For this review, take the finished solid that the model builds, in its own axes (mm). A direction names the side the tool comes from. Give positions to 0.01 mm unless a question says otherwise; leave off trailing zeros. Use a Markdown table: item, result. Add a question column.
1) Machinability: for faces 1 (the face through (6.35, 2, 2)), 2 (the face through (9.525, 0, 2)), which of the approach directions +Z, -Z, +X, -X, +Y, -Y give a long, thin tool a straight path to every point of the face, cutting with its end or side? Answer none if there is none.
2) Clearance check with flat-ended pins moving along their axes: P1, Ø10, axis at x = 4.5, y = 3.5, coming from the +Z side; P2, Ø2, axis at x = -4, z = 27.5, coming from the +Y side; P3, Ø6, axis at y = 7, z = 43, coming from the -X side; P4, Ø5, axis at y = -3, z = -22, coming from the -X side. State where each tip first meets the part, or that it passes through.
3) Wall thickness on L1, parallel to X at y = -7.8, z = 82.55 (3 decimals); L2, parallel to Y at x = 8.1, z = 82.55 (3 decimals); L3, parallel to X at y = -1.5, z = -38.5 (3 decimals): over which ranges is each line inside the solid? List them lowest first.
```python
from build123d import *

# Parameters (mm, degrees)
BOSS_EXTRUDE1_DEPTH          = 146.05
F_18_0_1695_DIAMETER_HOLE1_D = 4.3053
MIRROR2_COPY_1_D             = 4.3053
SKETCH19_W                   = 2.15265
SKETCH19_H                   = 3.175


with BuildPart() as part:
    # Sketch2 → Boss-Extrude1 (new, symmetric)
    with BuildSketch(Plane.XY):
        with BuildLine():
            Line((-9.525, -9.525), (9.525, -9.525))
            Line((9.525, -9.525), (9.525, 9.525))
            Line((9.525, 9.525), (7.9375, 9.525))
            ThreePointArc((7.9375, 9.525), (6.814967985, 9.060032015), (6.35, 7.9375))
            Line((6.35, 7.9375), (6.35, -3.175))
            ThreePointArc((6.35, -3.175), (5.42006403, -5.42006403), (3.175, -6.35))
            Line((3.175, -6.35), (-7.9375, -6.35))
            ThreePointArc((-7.9375, -6.35), (-9.060032015, -6.814967985), (-9.525, -7.9375))
            Line((-9.525, -7.9375), (-9.525, -9.525))
        make_face()
    extrude(amount=BOSS_EXTRUDE1_DEPTH, both=True)

    # #18 (0.1695) Diameter Hole1 (through all)
    with Locations(Plane.ZY.offset(-6.35)):
        with Locations((-95.25, 3.175), (-82.55, 3.175)):
            f_18_0_1695_diameter_hole1 = Hole(F_18_0_1695_DIAMETER_HOLE1_D / 2)

    # Mirror1: #18 (0.1695) Diameter Hole1 across plane
    add(f_18_0_1695_diameter_hole1.mirror(Plane(origin=(0, 0, 0), x_dir=(0, 0, 1), z_dir=(0.7071067811865477, 0.7071067811865475, 0))), mode=Mode.SUBTRACT)

    # Mirror2: #18 (0.1695) Diameter Hole1 across plane
    add(f_18_0_1695_diameter_hole1.mirror(Plane.XY), mode=Mode.SUBTRACT)

    # Mirror2 copy 1 (through all)
    with Locations(Plane(origin=(0, -6.35, 0), x_dir=(0, 0, -1), z_dir=(0, 1, 0))):
        with Locations((-95.25, 3.175), (-82.55, 3.175)):
            Hole(MIRROR2_COPY_1_D / 2)

    # Sketch19 → #8 Clearance Hole1 (revolve, cut)
    with BuildSketch(Plane(origin=(1.5875, -6.35, -134.9375), x_dir=(0, 0, 1), z_dir=(1, 0, 0))):
        with Locations((1.076325, 1.5875)):
            Rectangle(SKETCH19_W, SKETCH19_H)
    revolve(axis=Axis((1.5875, 0, -134.9375), (0, -1, 0)), mode=Mode.SUBTRACT)


solid = part.part
```
Checked values:
| question | item | result |
|---|---|---|
| 1 | face 1 | +Z, -Z, -X, +Y |
| 1 | face 2 | +Z, -Z, +X, +Y, -Y |
| 2 | P1 | z = 146.05 |
| 2 | P2 | y = -6.35 |
| 2 | P3 | x = 6.35 |
| 2 | P4 | x = 5.34 |
| 3 | L1 | -9.519 to -5.328, -1.022 to 9.525 |
| 3 | L2 | -9.525 to 1.022, 5.328 to 9.525 |
| 3 | L3 | 6.35 to 9.525 |
